Part model, mm, in its own coordinate system. Round coordinates to 2 decimals unless told otherwise and drop trailing zeros. Write each loop counter-clockwise with the first axis right and the second up, starting at its lowest first coordinate (ties: lowest second). Pieces come first, ordered by that corner, then holes. Notation, with made-up numbers: M 82,-31.5 L 109,-31.5 A15 cw 109,-12.5 Z; hole C 46,47 d10. An arc over 180 degrees is marked long. Use a Markdown table: item, result. Add a question column.
1) Slice it at B-B on x = -12.7. Write the cut outline in (y, z) (3 decimals).
2) Slice it at A-A on z = 63.5. Write the cut outline in (x, y) (3 decimals).
3) Wall check: probe 1 along X at (y, z) = (0.9, 63.5) (3 decimals); probe 2 along Z at (x, y) = (-114.3, 0.8) (3 decimals); probe 3 along Z at (x, y) = (-113, 2.45). Give the ranges that are in metal, low to high.
4) Two-plate mould, pull along Z, no slides. Class faces 1 (the face through (-45.617, 1.565, 30.805)), 2 (the face through (-64, 2, 76.2)), 3 (the face through (-63, 3.175, 39)): released by +Z, released by -Z, zero draft, split by the parting line, or undercut.
5) Slice it at C-C on y = 0.5. Give the number of separate pieces and of enclosed holes in the cut face, plus the area to 3 significant figures.
Autodesk Inventor part; units mm, degrees
ref_plane "YZ Plane" through (0, 0, 0) normal (1, 0, 0) x (0, 1, 0)
ref_plane "XZ Plane" through (0, 0, 0) normal (0, 1, 0) x (-1, 0, 0)
ref_plane "XY Plane" through (0, 0, 0) normal (0, 0, 1) x (1, 0, 0)
sketch "Sketch1" plane through (0, 0, 0) normal (0, 1, 0) x (-1, 0, 0)
  line L0 (0, 0) -> (127, 0)
  line L1 (127, 0) -> (127, 76.2)
  line L2 (127, 76.2) -> (0, 76.2)
  line L3 (0, 76.2) -> (0, 0)
  dimension "d0" = 76.2
  dimension "d2" = 127
extrude "Extrusion1" add sketch "Sketch1" along normal blind 3.175
sketch "Sketch2" plane through (0, 3.175, 0) normal (0, 1, 0) x (1, 0, 0)
  line L0 (0, 0) -> (-127, 0)
  line L1 (-127, 0) -> (-127, -76.2)
  line L2 (-127, -76.2) -> (0, -76.2)
  line L3 (0, -76.2) -> (0, 0)
  point P0 (-114.3, -12.7)
  point P1 (-114.3, -63.5)
  point P2 (-12.7, -63.5)
  point P3 (-12.7, -12.7)
  dimension "d5" = 12.7
  dimension "d6" = 12.7
  dimension "d7" = 12.7
  dimension "d8" = 12.7
  dimension "d9" = 12.7
  dimension "d10" = 12.7
  dimension "d11" = 12.7
  dimension "d12" = 12.7
  dimension "d13" = 50.8
  dimension "d14" = 101.6
  dimension "d15" = 50.8
hole "Hole1" at (-114.3, 3.175, 12.7) at (-114.3, 3.175, 63.5) at (-12.7, 3.175, 63.5) at (-12.7, 3.175, 12.7) direction (0, -1, 0) diameter 6.35 end through all
sketch "Sketch3" plane through (0, 3.175, 0) normal (0, 1, 0) x (1, 0, 0)
  line L0 (-127, 0) -> (-127, -76.2)
  line L1 (-127, -76.2) -> (0, -76.2)
  line L2 (0, -76.2) -> (0, 0)
  point P0 (-79.4512, -52.3748)
  point P1 (-47.5488, -52.3748)
  point P2 (-79.4512, -33.3248)
  point P3 (-47.5488, -33.3248)
  dimension "d23" = 47.5488
  dimension "d24" = 47.5488
  dimension "d25" = 47.5488
  dimension "d26" = 47.5488
  dimension "d27" = 19.05
  dimension "d28" = 19.05
  dimension "d29" = 23.8252
  dimension "d30" = 23.8252
hole "Hole2" at (-79.4512, 3.175, 52.3748) at (-47.5488, 3.175, 52.3748) at (-79.4512, 3.175, 33.3248) at (-47.5488, 3.175, 33.3248) direction (0, -1, 0) diameter 6.35 end through all
properties part number "CylinderPlate" material "Aluminum 6061"
Entries:
| question | item | result |
|---|---|---|
| 1 | outline | M 0,0 L 3.175,0 L 3.175,9.525 L 0,9.525 Z; M 0,15.875 L 3.175,15.875 L 3.175,60.325 L 0,60.325 Z; M 0,66.675 L 3.175,66.675 L 3.175,76.2 L 0,76.2 Z |
| 2 | outline | M -127,0 L -117.475,0 L -117.475,3.175 L -127,3.175 Z; M -111.125,0 L -15.875,0 L -15.875,3.175 L -111.125,3.175 Z; M -9.525,0 L 0,0 L 0,3.175 L -9.525,3.175 Z |
| 3 | probe 1 | x = -127 to -117.475, -111.125 to -15.875, -9.525 to 0 |
| 3 | probe 2 | z = 0 to 9.525, 15.875 to 60.325, 66.675 to 76.2 |
| 3 | probe 3 | z = 0 to 9.8, 15.6 to 60.6, 66.4 to 76.2 |
| 4 | face 1 | undercut |
| 4 | face 2 | released by +Z |
| 4 | face 3 | zero draft |
| 5 | separate pieces | 1 |
| 5 | enclosed holes | 8 |
| 5 | area | 9,420 mm^2 |
